Job drawing, mm, ordinate dimensions from the low corner. One solid piece. A direction names the side the tool comes from. Round coordinates to 2 decimals unless told otherwise and drop trailing zeros. Write each loop counter-clockwise with the first axis right and the second up, starting at its lowest first coordinate (ties: lowest second). Pieces come first, ordered by that corner, then holes. Notation, with made-up numbers: M 81.5,73 L 121.5,73 A23 cw 121.5,89 Z; hole C -18,17 d11. An arc over 180 degrees is marked long. Answer as a JSON object with one key per item and string values. Group by question number.
1. Which spindle directions (+Z, -Z, +X, -X, +Y, -Y) get a long thin tool onto all of the face, cutting with end or side? Do the marked faces 1, 2, 3 and 4. Say none if no direction does.
2. Drop flat-ended pins along their axis: pin 1 (6 mm diameter, centred on x = 10.5, z = 32.5, fed in from +Y); pin 2 (3 mm diameter, centred on x = 3.725, z = 3.725, fed in from +Y); pin 3 (3.5 mm diameter, centred on x = 37.5, y = 18, fed in from -Z) (3 decimals); pin 4 (7 mm diameter, centred on y = 12, z = 24.5, fed in from -X). Give the stop position or say it passes through.
3. Band-saw the part on B-B, the plane x = 35. Write the cut outline in (y, z) (3 decimals), plus the area to 3 significant figures.
4. Band-saw the part on D-D, the plane y = 24.75. Write the cut outline in (x, z) (3 decimals).
5. Band-saw the part on C-C, the plane z = 33. Write the cut outline in (x, y).
6. Band-saw the part on A-A, the plane x = 40. Write the cut outline in (y, z) (3 decimals).
7. Drill centre lines: line 1 (Z direction, x = 39, y = 15.75) (3 decimals); line 2 (X direction, y = 13.25, z = 11.5); line 3 (Y direction, x = 4, z = 18). Where is each one in solid material? Low to high. Write a range as from..to.
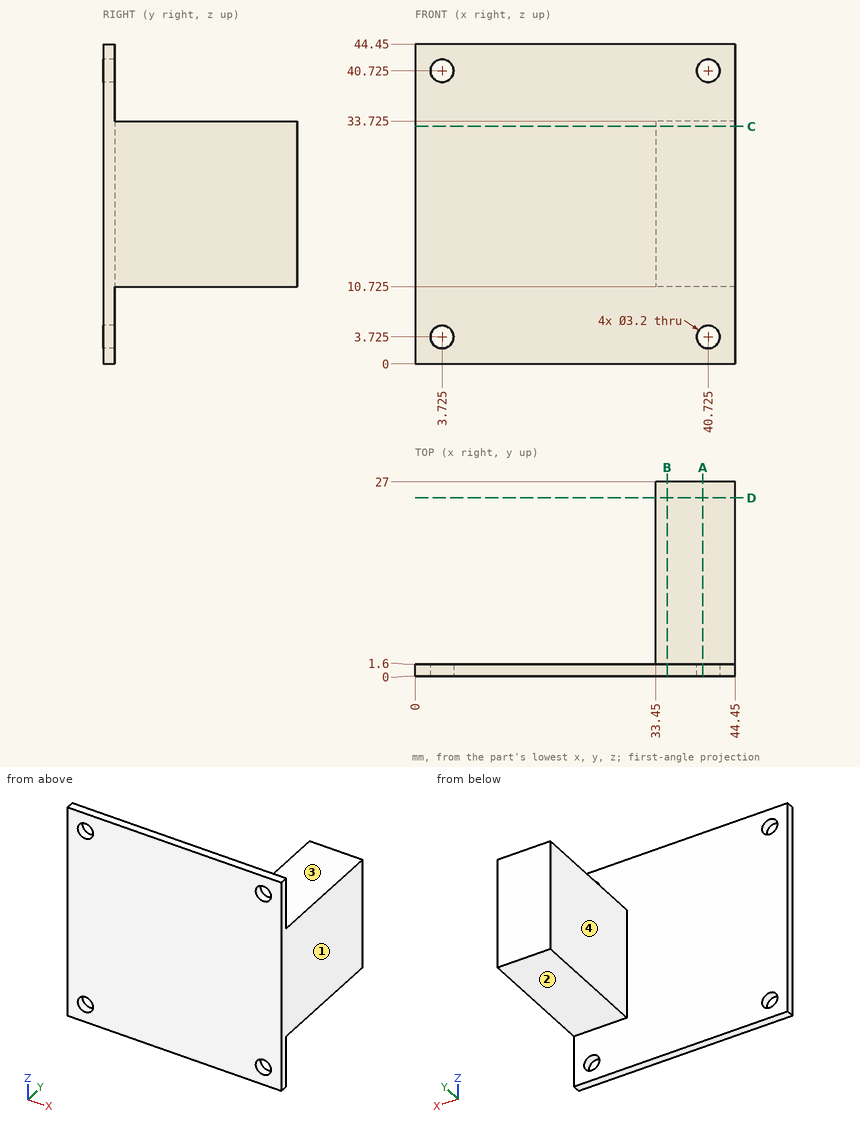
Worked answers:
{
 "1": {"face 1": "+Z, -Z, +X, +Y, -Y", "face 2": "-Z, +X, -X, +Y", "face 3": "+Z, +X, -X, +Y", "face 4": "+Z, -Z, -X, +Y"},
 "2": {"pin 1": "stops at y = 1.6", "pin 2": "passes through", "pin 3": "stops at z = 10.725", "pin 4": "stops at x = 33.45"},
 "3": {"outline": "M 0,0 L 1.6,0 L 1.6,10.725 L 27,10.725 L 27,33.725 L 1.6,33.725 L 1.6,44.45 L 0,44.45 Z", "area": "655 mm^2"},
 "4": {"outline": "M 33.45,10.725 L 44.45,10.725 L 44.45,33.725 L 33.45,33.725 Z"},
 "5": {"outline": "M 0,0 L 44.45,0 L 44.45,27 L 33.45,27 L 33.45,1.6 L 0,1.6 Z"},
 "6": {"outline": "M 0,0 L 1.6,0 L 1.6,2.299 L 0,2.299 Z; M 0,5.151 L 1.6,5.151 L 1.6,10.725 L 27,10.725 L 27,33.725 L 1.6,33.725 L 1.6,39.299 L 0,39.299 Z; M 0,42.151 L 1.6,42.151 L 1.6,44.45 L 0,44.45 Z"},
 "7": {"line 1": "z = 10.725..33.725", "line 2": "x = 33.45..44.45", "line 3": "y = 0..1.6"}
}
